Part print with two shaded views. Sizes in mm from the minimum x, y, z corner. A direction names the side the tool comes from. Round coordinates to 2 decimals unless told otherwise and drop trailing zeros. Order: outer loops, then holes, each group sorted by start corner. A loop starts at its lowest first (then second) coordinate and runs counter-clockwise, first axis right, second up. Notation, with made-up numbers: (10.5, -24.5) -> (60.5, -24.5) arc R15 cw to (60.5, -15.5) -> close; hole circle Ø5 at (58, 85). An arc over 180 degrees is marked (long way). Answer as a JSON object with one key per item and string values.
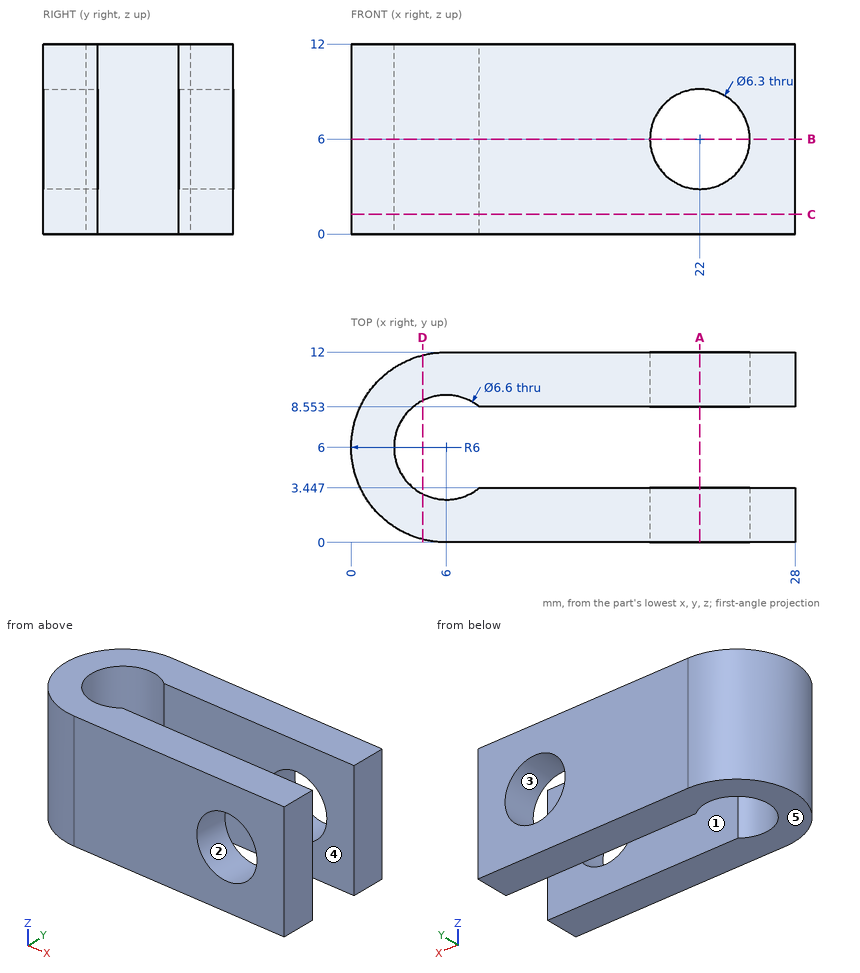
1) Probe L1, parallel to Y at x = 18, z = 0.5; L2, parallel to Y at x = 6, z = 5.25; L3, parallel to Z at x = 22, y = 2.55. List the from-to ranges inside material, lowest first. Write a range as from..to.
Checked values:
{"L1": "y = 0..3.45, 8.55..12", "L2": "y = 0..2.7, 9.3..12", "L3": "z = 0..2.85, 9.15..12"}
2) Flat gauge pin, fed straight in: pin 1 Ø5 at (y, z) = (10.5, 9) entering from -X. Where does the tip first touch, or does it go through?
Checked values:
{"pin 1": "stops at x = 0.34"}
3) Cut at D-D, the plane x = 4.5. Give the cut face in (y, z).
Checked values:
{"outline": "(0.19, 0) -> (3.06, 0) -> (3.06, 12) -> (0.19, 12) -> close; (8.94, 0) -> (11.81, 0) -> (11.81, 12) -> (8.94, 12) -> close"}
4) Pull direction Z, two halves, no side cores. Call the marked faces 3, 4 and 5: pulls with the +Z half, pulls with the -Z half, needs draft (parallel to the pull), parting line crosses it, or undercut.
Checked values:
{"face 3": "undercut", "face 4": "needs draft", "face 5": "pulls with the -Z half"}
5) Which spindle directions (+Z, -Z, +X, -X, +Y, -Y) get a long thin tool onto all of the face, cutting with end or side? Do the marked faces 1 and 2. Say none if no direction does.
Checked values:
{"face 1": "+Z, -Z, +X", "face 2": "+Y, -Y"}
6) Cut at C-C, the plane z = 1.25. Give the cut face in (x, y), plus the area to 3 significant figures.
Checked values:
{"outline": "(6, 0) -> (28, 0) -> (28, 3.45) -> (8.09, 3.45) arc R3.3 cw (long way) to (8.09, 8.55) -> (28, 8.55) -> (28, 12) -> (6, 12) arc R6 ccw to start", "area": "189 mm²"}
7) Cut at A-A, the plane x = 22. Give the cut face in (y, z).
Checked values:
{"outline": "(0, 0) -> (3.45, 0) -> (3.45, 2.85) -> (0, 2.85) -> close; (0, 9.15) -> (3.45, 9.15) -> (3.45, 12) -> (0, 12) -> close; (8.55, 0) -> (12, 0) -> (12, 2.85) -> (8.55, 2.85) -> close; (8.55, 9.15) -> (12, 9.15) -> (12, 12) -> (8.55, 12) -> close"}
8) Cut at B-B, the plane z = 6. Give the cut face in (x, y).
Checked values:
{"outline": "(6, 0) -> (18.85, 0) -> (18.85, 3.45) -> (8.09, 3.45) arc R3.3 cw (long way) to (8.09, 8.55) -> (18.85, 8.55) -> (18.85, 12) -> (6, 12) arc R6 ccw to start; (25.15, 0) -> (28, 0) -> (28, 3.45) -> (25.15, 3.45) -> close; (25.15, 8.55) -> (28, 8.55) -> (28, 12) -> (25.15, 12) -> close"}
